```python
from build123d import *

# Parameters (mm, degrees)
F1_DEPTH = 5


with BuildPart() as f1:
    # F0 (on Front) → F1 (new body, symmetric)
    with BuildSketch(Plane.XZ):
        with BuildLine():
            Line((5, 0), (0, 0))
            Line((0, 0), (-0.016378, 0))
            Line((-0.016378, 0), (-0.617307, -0.397922))
            Line((-0.617307, -0.397922), (0, 0.353466))
            Line((0, 0.353466), (0, 5.71834))
            Line((0, 5.71834), (-0.456822, 6.408219))
            Line((-0.456822, 6.408219), (0.283503, 5.8))
            Line((0.283503, 5.8), (5, 5.8))
            ThreePointArc((5, 5.8), (4.416528, 7.2119), (3.00655, 7.8))
            Line((3.00655, 7.8), (-1.5, 7.8))
            ThreePointArc((-1.5, 7.8), (-1.853553, 7.653553), (-2, 7.3))
            Line((-2, 7.3), (-2, -1.7))
            ThreePointArc((-2, -1.7), (-1.853553, -2.053553), (-1.5, -2.2))
            Line((-1.5, -2.2), (3.00655, -2.2))
            ThreePointArc((3.00655, -2.2), (4.427511, -1.484406), (5, 0))
        make_face()
    extrude(amount=F1_DEPTH, both=True)


solid = f1.part
```
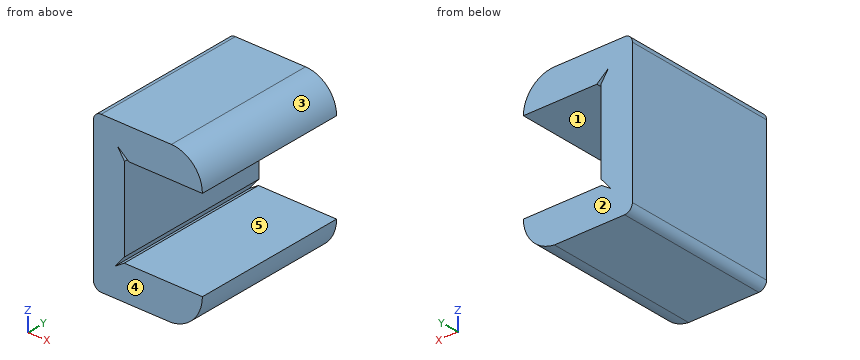
Here's how the part is built. I have some questions about the finished solid (model axes, mm). Face numbers are marked on the shaded views. A direction names the side the tool comes from. Give positions to 0.01 mm unless a question says otherwise; leave off trailing zeros. Order: outer loops, then holes, each group sorted by start corner. A loop starts at its lowest first (then second) coordinate and runs counter-clockwise, first axis right, second up. Notation, with made-up numbers: (-32, 37) - (-10, 37) arc R22 ccw to (-10, 62) - close; hole circle Ø10 at (59, 82.25). An arc over 180 degrees is marked (long way). Answer as a JSON object with one key per item and string values. Group by question number.
Item 1: Please list where these lines run through material, in increasing order: probe 1 along Z at (x, y) = (1.5, 2.25); probe 2 along X at (y, z) = (3.5, 4.25); probe 3 along Z at (x, y) = (4, 2.75).
Item 2: If we section it at B-B on y = -0.75: Please give me the cut outline in (x, z), and give its area (3 significant figures).
Item 3: If we mould it in two halves opening along Z, with no side actions, what happens to the marked faces 3, 4 and 5? For each: pulls with the +Z half, pulls with the -Z half, needs draft (parallel to the pull), parting line crosses it, or undercut.
Item 4: If we section it at D-D on x = 4.5: Please give me the cut outline in (y, z).
Item 5: If we section it at C-C on z = 3.5: Please give me the cut outline in (x, y), and give its area (3 significant figures).
Item 6: For P1, Ø2, axis at y = -0.5, z = 4, coming from the +X side; P2, Ø4, axis at x = 3.5, y = 1.5, coming from the -Z side, each with a flat end and sliding along its axis, tell me the tip position at first contact or that it passes through.
Item 7: Which directions (+Z, -Z, +X, -X, +Y, -Y) give clear straight access to the entire face, cutting with the end or side of a thin tool? Please do the marked faces 1 and 2.
Item 8: If we section it at A-A on x = 2.5: Please give me the cut outline in (y, z).
Result set:
{
 "1": {"probe 1": "-2.2 to 0, 5.8 to 7.8", "probe 2": "-2 to 0", "probe 3": "-1.85 to 0, 5.8 to 7.53"},
 "2": {"outline": "(-2, -1.7) arc R0.5 ccw to (-1.5, -2.2) - (3.01, -2.2) arc R2.21 ccw to (5, 0) - (-0.02, 0) - (-0.62, -0.4) - (0, 0.35) - (0, 5.72) - (-0.46, 6.41) - (0.28, 5.8) - (5, 5.8) arc R2 ccw to (3.01, 7.8) - (-1.5, 7.8) arc R0.5 ccw to (-2, 7.3) - close", "area": "38.8 mm²"},
 "3": {"face 3": "pulls with the +Z half", "face 4": "needs draft", "face 5": "undercut"},
 "4": {"outline": "(-5, -1.4) - (5, -1.4) - (5, 0) - (-5, 0) - close; (-5, 5.8) - (5, 5.8) - (5, 7.12) - (-5, 7.12) - close"},
 "5": {"outline": "(-2, -5) - (0, -5) - (0, 5) - (-2, 5) - close", "area": "20.0 mm²"},
 "6": {"P1": "x = 0", "P2": "z = -2.2"},
 "7": {"face 1": "+X, +Y, -Y", "face 2": "+Z, -Z, +X, -X, +Y"},
 "8": {"outline": "(-5, -2.2) - (5, -2.2) - (5, 0) - (-5, 0) - close; (-5, 5.8) - (5, 5.8) - (5, 7.8) - (-5, 7.8) - close"}
}
